Geometry check sheet. Reference: the model listing, model coordinates, mm. A direction names the side the tool comes from. Give positions to 0.01 mm unless a question says otherwise; leave off trailing zeros. Loops run counter-clockwise (first coordinate to the right, second up) from the corner with the lowest first, then second, coordinate; pieces in that order, holes last. Notation, with made-up numbers: (57.5, 13.25) -> (86.5, 13.25) arc R7 cw to (86.5, 23.25) -> close; hole circle Ø2 at (76.25, -37). An arc over 180 degrees is marked (long way). Answer as a JSON object with one key per item and string values.
from build123d import *

# Parameters (mm, degrees)
F1_DEPTH  = 508
F3_DEPTH  = 406.4
F4_T      = -12.7
F6_DEPTH  = 508.001
F8_DEPTH  = 25.4
F10_DEPTH = 25.4
F11_W     = 508
F11_H     = 431.8
F12_DEPTH = 3


with BuildPart() as f1:
    # F0 (on Front) → F1 (new body)
    with BuildSketch(Plane.XZ):
        Polygon((-228.6, 155.0921710968), (-228.6, -251.3078289032), (279.4, -251.3078289032), (279.4, 155.0921710968), (228.6, 256.6921710968), (-177.8, 256.6921710968), align=None)
    extrude(amount=F1_DEPTH)

    # F2 (on face) → F3 (join)
    with BuildSketch(Plane(origin=(0, 0, 0), x_dir=(-1, 0, 0), z_dir=(0, 1, 0))):
        Polygon((-279.4, 409.0921710968), (-279.4, -251.3078289032), (228.6, -251.3078289032), (228.6, 409.0921710968), (177.8, 510.6921710968), (-228.6, 510.6921710968), align=None)
    extrude(amount=F3_DEPTH)

    # F4
    f4_openings = [f1.faces().sort_by_distance(p)[0] for p in [
        (25.4, -50.8, -251.307829),
        (25.4, 406.4, 125.00118),
    ]]
    offset(amount=F4_T, openings=f4_openings, kind=Kind.INTERSECTION)

    # F5 (on face) → F6 (cut, through all)
    with BuildSketch(Plane.YZ.offset(279.4)):
        with BuildLine():
            Line((406.4, 180.4921710968), (406.4, 383.6921710968))
            Line((406.4, 383.6921710968), (76.2, 383.6921710968))
            ThreePointArc((76.2, 383.6921710968), (58.2394877579, 376.2526833389), (50.8, 358.2921710968))
            Line((50.8, 358.2921710968), (50.8, 205.8921710968))
            ThreePointArc((50.8, 205.8921710968), (58.2394877579, 187.9316588547), (76.2, 180.4921710968))
            Line((76.2, 180.4921710968), (406.4, 180.4921710968))
        make_face()
    extrude(amount=-F6_DEPTH, mode=Mode.SUBTRACT)

    # F7 (on face) → F8 (cut)
    with BuildSketch(Plane.XZ.offset(508)):
        with BuildLine():
            Line((203.2, 104.2921710968), (-152.4, 104.2921710968))
            ThreePointArc((-152.4, 104.2921710968), (-170.3605122421, 96.8526833389), (-177.8, 78.8921710968))
            Line((-177.8, 78.8921710968), (-177.8, -175.1078289032))
            ThreePointArc((-177.8, -175.1078289032), (-170.3605122421, -193.0683411453), (-152.4, -200.5078289032))
            Line((-152.4, -200.5078289032), (203.2, -200.5078289032))
            ThreePointArc((203.2, -200.5078289032), (221.1605122421, -193.0683411453), (228.6, -175.1078289032))
            Line((228.6, -175.1078289032), (228.6, 78.8921710968))
            ThreePointArc((228.6, 78.8921710968), (221.1605122421, 96.8526833389), (203.2, 104.2921710968))
        make_face()
    extrude(amount=-F8_DEPTH, mode=Mode.SUBTRACT)

    # F9 (on face) → F10 (cut)
    with BuildSketch(Plane.XZ):
        with BuildLine():
            ThreePointArc((-177.8, 332.8921710968), (-170.3605122421, 314.9316588547), (-152.4, 307.4921710968))
            Line((-152.4, 307.4921710968), (-50.8, 307.4921710968))
            ThreePointArc((-50.8, 307.4921710968), (-32.8394877579, 314.9316588547), (-25.4, 332.8921710968))
            Line((-25.4, 332.8921710968), (-25.4, 434.4921710968))
            ThreePointArc((-25.4, 434.4921710968), (-32.8394877579, 452.4526833389), (-50.8, 459.8921710968))
            Line((-50.8, 459.8921710968), (-130.7058100573, 459.8921710968))
            ThreePointArc((-130.7058100573, 459.8921710968), (-144.0593803051, 456.0987016289), (-153.4242607087, 445.8513964225))
            Line((-153.4242607087, 445.8513964225), (-175.1184506514, 402.463016537))
            ThreePointArc((-175.1184506514, 402.463016537), (-177.1205243325, 396.9395153932), (-177.8, 391.1037912113))
            Line((-177.8, 391.1037912113), (-177.8, 332.8921710968))
        make_face()
        with BuildLine():
            ThreePointArc((101.6, 459.8921710968), (83.6394877579, 452.4526833389), (76.2, 434.4921710968))
            Line((76.2, 434.4921710968), (76.2, 332.8921710968))
            ThreePointArc((76.2, 332.8921710968), (83.6394877579, 314.9316588547), (101.6, 307.4921710968))
            Line((101.6, 307.4921710968), (203.2, 307.4921710968))
            ThreePointArc((203.2, 307.4921710968), (221.1605122421, 314.9316588547), (228.6, 332.8921710968))
            Line((228.6, 332.8921710968), (228.6, 391.1037912113))
            ThreePointArc((228.6, 391.1037912113), (227.9205243325, 396.9395153932), (225.9184506514, 402.463016537))
            Line((225.9184506514, 402.463016537), (204.2242607087, 445.8513964225))
            ThreePointArc((204.2242607087, 445.8513964225), (194.8593803051, 456.0987016289), (181.5058100573, 459.8921710968))
            Line((181.5058100573, 459.8921710968), (101.6, 459.8921710968))
        make_face()
    extrude(amount=-F10_DEPTH, mode=Mode.SUBTRACT)

    # F11 (on face) → F12 (join)
    with BuildSketch(Plane(origin=(0, 406.4, 0), x_dir=(-1, 0, 0), z_dir=(0, 1, 0))):
        with Locations((-25.4, -35.4078289032)):
            Rectangle(F11_W, F11_H)
    extrude(amount=-F12_DEPTH)


solid = f1.part
1) Section check A-A on z = 346. Record the cut outline in (x, y), plus the area to 3 significant figures.
Geometry check:
{"outline": "(-228.6, 0) -> (-177.8, 0) -> (-177.8, 12.7) -> (-215.9, 12.7) -> (-215.9, 50.8) -> (-228.6, 50.8) -> close; (-25.4, 0) -> (76.2, 0) -> (76.2, 12.7) -> (-25.4, 12.7) -> close; (228.6, 0) -> (279.4, 0) -> (279.4, 50.8) -> (266.7, 50.8) -> (266.7, 12.7) -> (228.6, 12.7) -> close", "area": "3,550 mm2"}
2) Section check D-D on z = -65.5. Record the cut outline in (x, y).
Geometry check:
{"outline": "(-228.6, -508) -> (-177.8, -508) -> (-177.8, -495.3) -> (-215.9, -495.3) -> (-215.9, 403.4) -> (266.7, 403.4) -> (266.7, -495.3) -> (228.6, -495.3) -> (228.6, -508) -> (279.4, -508) -> (279.4, 406.4) -> (-228.6, 406.4) -> close"}
3) Depth check by flat-ended pin: P1, Ø4, axis at x = -223, z = 283, coming from the +Y side; P2, Ø10, axis at x = 40, y = 223, coming from the -Z side; P3, Ø6.5, axis at x = -77.5, y = 5, coming from the -Z side. Enter the tip coordinate at first touch or a pass-through.
Geometry check:
{"P1": "stops at y = 50.8", "P2": "stops at z = 497.99", "P3": "stops at z = 243.99"}
4) Material ranges on line 1 along X through (y, z) = (-390.5, -70); line 2 along Y through (x, z) = (-23.5, 126.5); line 3 along Z through (x, y) = (18, -142), recorded low to high. Write a range as from..to.
Geometry check:
{"line 1": "x = -228.6..-215.9, 266.7..279.4", "line 2": "y = -508..-495.3, 403.4..406.4", "line 3": "z = 243.99..256.69"}
5) Tool access check on faces 4 (the face through (-222.16, 58.44, 376.45)), 5 (the face through (-33.038, 6.261, 314.735)), 6 (the face through (-170.16, -501.74, 97.05)), 7 (the face through (-192.6, -237.74, 198.69)), 8 (the face through (243.4, 206.79, 452.69)). Record the directions out of +Z, -Z, +X, -X, +Y, -Y that give a thin tool (end or side, any length) a straight path to the whole face; none if there is none.
Geometry check:
{"face 4": "+X, -X, +Y", "face 5": "+Y, -Y", "face 6": "-Y", "face 7": "-Z", "face 8": "-Z, +Y"}
6) Section check C-C on x = 25. Record the cut outline in (y, z), plus the area to 3 significant figures.
Geometry check:
{"outline": "(-508, -251.31) -> (-495.3, -251.31) -> (-495.3, -200.51) -> (-508, -200.51) -> close; (-508, 104.29) -> (-495.3, 104.29) -> (-495.3, 243.99) -> (12.7, 243.99) -> (12.7, 497.99) -> (406.4, 497.99) -> (406.4, 510.69) -> (0, 510.69) -> (0, 256.69) -> (-508, 256.69) -> close; (403.4, -251.31) -> (406.4, -251.31) -> (406.4, 180.49) -> (403.4, 180.49) -> close", "area": "18,600 mm2"}
7) Draft check along X on faces 1 (the face through (28, -238, 243.992)), 2 (the face through (279.4, -57, 10)), 3 (the face through (27, 406.4, 499)). Enter one of: pulls with the +X half, pulls with the -X half, needs draft (parallel to the pull), parting line crosses it, or undercut.
Geometry check:
{"face 1": "undercut", "face 2": "pulls with the +X half", "face 3": "needs draft"}
8) Section check B-B on y = 93.5. Record the cut outline in (x, z).
Geometry check:
{"outline": "(-228.6, -251.31) -> (-215.9, -251.31) -> (-215.9, 180.49) -> (-228.6, 180.49) -> close; (-228.6, 383.69) -> (-215.9, 383.69) -> (-215.9, 406.09) -> (-169.95, 497.99) -> (220.75, 497.99) -> (266.7, 406.09) -> (266.7, 383.69) -> (279.4, 383.69) -> (279.4, 409.09) -> (228.6, 510.69) -> (-177.8, 510.69) -> (-228.6, 409.09) -> close; (266.7, -251.31) -> (279.4, -251.31) -> (279.4, 180.49) -> (266.7, 180.49) -> close"}
